Part model, mm, in its own coordinate system. A direction names the side the tool comes from. Round coordinates to 2 decimals unless told otherwise and drop trailing zeros. Loops run counter-clockwise (first coordinate to the right, second up) from the corner with the lowest first, then second, coordinate; pieces in that order, holes last.
1) 3-axis set-ups, long thin cutter, end or side, ignore diameter. For faces 1 (the flat face through (-2.24, 9.51, 6.29)), 2 (the flat face through (9.593, 4.93, 1.956)), 3 (the flat face through (0, 5, -11)), 4 (the flat face through (-8.167, 4.93, 5.4)), 5 (the flat face through (5.4, 4.93, 8.167)): which of +Z, -Z, +X, -X, +Y, -Y reach the whole face in a straight line?
2) Band-saw the part on D-D, the plane x = 3. Write the cut outline in (y, z), then the cut area to 3 significant figures.
3) Band-saw the part on C-C, the plane x = 5.75. Write the cut outline in (y, z), then the cut area to 3 significant figures.
4) Mould opens along Z. For faces 6 (the cylindrical face through (-7.86, 4.93, -3.24)), 7 (the cylindrical face through (1.016, 4.684, -0.133)), 8 (the cylindrical face through (3.24, 4.93, -7.86)), 9 (the flat face through (11, 5, 0)) say: +Z half, -Z half, draft (parallel to the pull), parting line (faces both ways), or undercut.
5) Band-saw the part on B-B, the plane z = 0. Write the cut outline in (x, y) (3 decimals).
6) Drop a flat-ended pin along its axis: P1, Ø2.5, axis at x = 0, z = 0, coming from the +Y side (3 decimals). Give the stop position or say it passes through.
7) Probe line 1 (Z direction, x = -8.75, y = 0.75); line 2 (X direction, y = 2, z = 0) (3 decimals). List the from-to ranges inside material, lowest first.
from build123d import *

# Parameters (mm, degrees)
SKETCH1_R           = 1.025
BOSS_EXTRUDE1_DEPTH = 10
CUT_EXTRUDE1_DEPTH  = 1
CHAMFER1_SIZE       = 0.5


with BuildPart() as part:
    # Sketch1 → Boss-Extrude1 (new body)
    with BuildSketch(Plane(origin=(0, 0, 0), x_dir=(1, 0, 0), z_dir=(0, 1, 0))):
        with BuildLine():
            Line((-1.5, 11), (1.5, 11))
            Line((1.5, 11), (2.425924848, 8.146464793))
            ThreePointArc((2.425924848, 8.146464793), (3.252809175, 7.852976026), (4.045032587, 7.475808409))
            Line((4.045032587, 7.475808409), (6.717514421, 8.838834765))
            Line((6.717514421, 8.838834765), (8.838834765, 6.717514421))
            Line((8.838834765, 6.717514421), (7.475808409, 4.045032587))
            ThreePointArc((7.475808409, 4.045032587), (7.852976026, 3.252809175), (8.146464793, 2.425924848))
            Line((8.146464793, 2.425924848), (11, 1.5))
            Line((11, 1.5), (11, -1.5))
            Line((11, -1.5), (8.146464793, -2.425924848))
            ThreePointArc((8.146464793, -2.425924848), (7.852976026, -3.252809175), (7.475808409, -4.045032587))
            Line((7.475808409, -4.045032587), (8.838834765, -6.717514421))
            Line((8.838834765, -6.717514421), (6.717514421, -8.838834765))
            Line((6.717514421, -8.838834765), (4.045032587, -7.475808409))
            ThreePointArc((4.045032587, -7.475808409), (3.252809175, -7.852976026), (2.425924848, -8.146464793))
            Line((2.425924848, -8.146464793), (1.5, -11))
            Line((1.5, -11), (-1.5, -11))
            Line((-1.5, -11), (-2.425924848, -8.146464793))
            ThreePointArc((-2.425924848, -8.146464793), (-3.252809175, -7.852976026), (-4.045032587, -7.475808409))
            Line((-4.045032587, -7.475808409), (-6.717514421, -8.838834765))
            Line((-6.717514421, -8.838834765), (-8.838834765, -6.717514421))
            Line((-8.838834765, -6.717514421), (-7.475808409, -4.045032587))
            ThreePointArc((-7.475808409, -4.045032587), (-7.852976026, -3.252809175), (-8.146464793, -2.425924848))
            Line((-8.146464793, -2.425924848), (-11, -1.5))
            Line((-11, -1.5), (-11, 1.5))
            Line((-11, 1.5), (-8.146464793, 2.425924848))
            ThreePointArc((-8.146464793, 2.425924848), (-7.852976026, 3.252809175), (-7.475808409, 4.045032587))
            Line((-7.475808409, 4.045032587), (-8.838834765, 6.717514421))
            Line((-8.838834765, 6.717514421), (-6.717514421, 8.838834765))
            Line((-6.717514421, 8.838834765), (-4.045032587, 7.475808409))
            ThreePointArc((-4.045032587, 7.475808409), (-3.252809175, 7.852976026), (-2.425924848, 8.146464793))
            Line((-2.425924848, 8.146464793), (-1.5, 11))
        make_face()
        with Locations(Location((0, 0, 0), (0, 0, 270))):
            Circle(SKETCH1_R, mode=Mode.SUBTRACT)
    extrude(amount=BOSS_EXTRUDE1_DEPTH)

    # Sketch2 → Cut-Extrude1 (cut)
    with BuildSketch(Plane(origin=(0, 10, 0), x_dir=(1, 0, 0), z_dir=(0, 1, 0))):
        with BuildLine():
            Line((-0.67951288, -5.685173621), (-0.647962399, -5.449296217))
            add(Edge.make_bspline(
                [(-0.647962399, -5.449296217), (-0.618308174, -5.454820304), (-0.560284153, -5.465629209), (-0.476362431, -5.48984076), (-0.397731022, -5.521051701), (-0.323681884, -5.55793727), (-0.2551006, -5.601861634), (-0.191688594, -5.652375632), (-0.132801937, -5.708925264), (-0.0801525, -5.772097211), (-0.033306561, -5.838981745), (0.006196757, -5.909238602), (0.037797909, -5.981878785), (0.061604112, -6.057047051), (0.077052172, -6.134660608), (0.08492264, -6.214640896), (0.085830566, -6.29719701), (0.079775803, -6.352610008), (0.076697056, -6.380786602)],
                knots=[0, 0, 0, 0, 1.100859962, 2.154037817, 3.182825855, 4.185872747, 5.169851411, 6.150256119, 7.141625092, 8.14517181, 9.147774204, 10.119215176, 11.08276616, 12.034993632, 12.992414738, 13.96637616, 14.965935861, 16, 16, 16, 16], degree=3))
            add(Edge.make_bspline(
                [(0.076697056, -6.380786602), (0.072393378, -6.408440649), (0.063964293, -6.462603227), (0.04245955, -6.540444475), (0.015673176, -6.613601341), (-0.018163052, -6.681449321), (-0.057782709, -6.744623459), (-0.104369947, -6.802540115), (-0.156916189, -6.855759765), (-0.215482247, -6.903032984), (-0.277774366, -6.944150039), (-0.342035354, -6.979710839), (-0.408235726, -7.007659397), (-0.475930945, -7.029042638), (-0.545273153, -7.043093792), (-0.616231572, -7.049848725), (-0.688708826, -7.050812711), (-0.737134817, -7.045523091), (-0.76164429, -7.042845897)],
                knots=[0, 0, 0, 0, 1.125087727, 2.203570911, 3.242694659, 4.254840133, 5.247912274, 6.236956909, 7.238958616, 8.25110409, 9.25878367, 10.238550544, 11.20150929, 12.144591564, 13.090252789, 14.041833295, 15.008928189, 16, 16, 16, 16], degree=3))
            add(Edge.make_bspline(
                [(-0.76164429, -7.042845897), (-0.795911856, -7.037073204), (-0.863853491, -7.025627798), (-0.961802832, -6.992522173), (-1.055166763, -6.948613121), (-1.128556526, -6.900437931), (-1.18688245, -6.854457889), (-1.234181818, -6.813349399), (-1.285078121, -6.766197674), (-1.338253587, -6.711815369), (-1.395526889, -6.651708318), (-1.456041505, -6.585144653), (-1.519640402, -6.511855414), (-1.562672338, -6.460481627), (-1.584961598, -6.433871538)],
                knots=[0, 0, 0, 0, 1.188707215, 2.356826555, 3.52825813, 4.714611235, 5.354043377, 6.071637886, 6.860592227, 7.729914435, 8.676361207, 9.70450881, 10.811004006, 12, 12, 12, 12], degree=3))
            Line((-1.584961598, -6.433871538), (-2.164889482, -5.732248942))
            Line((-2.164889482, -5.732248942), (-2.316632271, -6.869067852))
            Line((-2.316632271, -6.869067852), (-2.55451288, -6.837517371))
            Line((-2.55451288, -6.837517371), (-2.331155508, -5.164841089))
            Line((-2.331155508, -5.164841089), (-1.440230027, -6.241563846))
            add(Edge.make_bspline(
                [(-1.440230027, -6.241563846), (-1.418649822, -6.267874505), (-1.377249469, -6.318349956), (-1.315768194, -6.38934036), (-1.259427886, -6.454151648), (-1.206885587, -6.511815526), (-1.158177578, -6.562464113), (-1.114045746, -6.606526292), (-1.073683056, -6.643345812), (-1.026325868, -6.683346431), (-0.967044732, -6.723557397), (-0.892856227, -6.760623309), (-0.81553634, -6.788990522), (-0.761683927, -6.797953641), (-0.734601021, -6.802461281)],
                knots=[0, 0, 0, 0, 1.32529596, 2.542502302, 3.657515733, 4.670000406, 5.580482446, 6.394245158, 7.098391746, 7.707758491, 8.807790529, 9.877823122, 10.932736443, 12, 12, 12, 12], degree=3))
            add(Edge.make_bspline(
                [(-0.734601021, -6.802461281), (-0.717426635, -6.80438222), (-0.68363806, -6.80816144), (-0.633127366, -6.806556794), (-0.583869632, -6.801558493), (-0.535919132, -6.790163413), (-0.489098591, -6.774099208), (-0.443345088, -6.752865521), (-0.398672819, -6.726802578), (-0.35592185, -6.695740886), (-0.315566891, -6.661189714), (-0.279504864, -6.622950363), (-0.247530448, -6.582201059), (-0.220631343, -6.538310443), (-0.197234923, -6.492062695), (-0.178790476, -6.442668271), (-0.164583049, -6.390524125), (-0.15900309, -6.354480024), (-0.15617554, -6.336215288)],
                knots=[0, 0, 0, 0, 1.002635519, 1.972567043, 2.928877794, 3.874508698, 4.828259305, 5.800176361, 6.799758996, 7.8278638, 8.866026664, 9.881245134, 10.876349012, 11.869324323, 12.866787948, 13.882608331, 14.927047686, 16, 16, 16, 16], degree=3))
            add(Edge.make_bspline(
                [(-0.15617554, -6.336215288), (-0.15395807, -6.316878514), (-0.149590127, -6.278789182), (-0.149692165, -6.222212083), (-0.155357805, -6.167410823), (-0.165690288, -6.114526465), (-0.181382515, -6.063304443), (-0.202439411, -6.014053189), (-0.229260456, -5.966903638), (-0.260809506, -5.921672896), (-0.297362541, -5.879390265), (-0.338000583, -5.839781192), (-0.384025516, -5.804833072), (-0.434318992, -5.773209858), (-0.489037939, -5.745030253), (-0.548513417, -5.721234969), (-0.612167638, -5.700363512), (-0.656711876, -5.690316446), (-0.67951288, -5.685173621)],
                knots=[0, 0, 0, 0, 1.003940432, 1.977549207, 2.912892054, 3.843939206, 4.754223491, 5.672869237, 6.602639779, 7.549185681, 8.514563016, 9.483432891, 10.472624027, 11.490954394, 12.546793215, 13.644379156, 14.7942207, 16, 16, 16, 16], degree=3))
        make_face()
    extrude(amount=-CUT_EXTRUDE1_DEPTH, mode=Mode.SUBTRACT)

    # Chamfer1
    chamfer1_edges = [part.edges().sort_by_distance(p)[0] for p in [
        (0, 10, -1.025),
    ]]
    chamfer(chamfer1_edges, length=CHAMFER1_SIZE)


solid = part.part
Reported:
1. face 1: +Y
1. face 2: +X, +Y, -Y
1. face 3: -Z, +X, -X, +Y, -Y
1. face 4: -X, +Y, -Y
1. face 5: +Z, +Y, -Y
2. outline: (0, -7.95) - (10, -7.95) - (10, 7.95) - (0, 7.95) - close
2. area: 159 mm2
3. outline: (0, -8.35) - (10, -8.35) - (10, 8.35) - (0, 8.35) - close
3. area: 167 mm2
4. face 6: undercut
4. face 7: undercut
4. face 8: -Z half
4. face 9: draft
5. outline: (-11, 0) - (-1.025, 0) - (-1.025, 9.5) - (-1.525, 10) - (-11, 10) - close; (1.025, 0) - (11, 0) - (11, 10) - (1.525, 10) - (1.025, 9.5) - close
6. P1: stops at y = 9.725
7. line 1: z = -6.81 to -6.54, -2.23 to 2.23, 6.54 to 6.81
7. line 2: x = -11 to -1.025, 1.025 to 11
